from build123d import *

# Parameters (mm, degrees)
BOSS_EXTRUDE1_DEPTH     = 70
CUT_EXTRUDE2_DEPTH      = 83.5
CUT_EXTRUDE2_DEPTH_BACK = 83.5


with BuildPart() as part:
    # Sketch1 → Boss-Extrude1 (new body)
    with BuildSketch(Plane(origin=(0, 0, 0), x_dir=(1, 0, 0), z_dir=(0, 1, 0))):
        Polygon((-42.5, 0), (42.5, 0), (42.5, 10), (41.5, 10), (41.5, 1), (-41.5, 1), (-41.5, 10), (-42.5, 10), align=None)
    extrude(amount=BOSS_EXTRUDE1_DEPTH)

    # Sketch2 → Cut-Extrude2 (cut, two sides: drawn at the far end of the back side and taken through both)
    with BuildSketch(Plane(origin=(0, 0, 0), x_dir=(0, 0, -1), z_dir=(1, 0, 0)).offset(-CUT_EXTRUDE2_DEPTH_BACK)):
        Polygon((1, 70), (10, 55), (10, 70), align=None)
    extrude(amount=CUT_EXTRUDE2_DEPTH + CUT_EXTRUDE2_DEPTH_BACK, mode=Mode.SUBTRACT)


solid = part.part
Geometry check sheet. Reference: the model listing, model coordinates, mm. A direction names the side the tool comes from. Round coordinates to 2 decimals unless told otherwise and drop trailing zeros. Write each loop counter-clockwise with the first axis right and the second up, starting at its lowest first coordinate (ties: lowest second). Pieces come first, ordered by that corner, then holes. Notation, with made-up numbers: (46, -9) -> (67, -9) arc R13 ccw to (67, 4) -> close; hole circle Ø3 at (88, 59.5). An arc over 180 degrees is marked (long way). One line per item, written item: value. Start each with the question number.
(1) Draft check along X on faces 1 (the flat face through (-42.5, 35, -5)), 2 (the flat face through (1, 35, -1)), 3 (the flat face through (41.99, 62.6, -5.44)). Enter one of: +X half, -X half, draft (parallel to the pull), parting line (faces both ways), or undercut.
(2) Access from +Z, -Z, +X, -X, +Y, -Y to the whole of each face (thin tool, end or side, straight path). Record for faces 4 (the flat face through (-1, 35, 0)), 5 (the flat face through (-41.5, 35, -5)).
(3) Cross-section at D-D, the plane z = -8.25. Record the cut outline in (x, y), and give its area (3 significant figures).
(4) Cross-section at B-B, the plane y = 51. Record the cut outline in (x, z).
(5) Scan lines: line 1 (X direction, y = 48.5, z = -7); line 2 (Z direction, x = -9.5, y = 33.5). Record each from-to range of solid material in increasing order. Write a range as [from, to].
(6) Go/stop test with a flat-tipped pin: pin 1 Ø6 at (x, y) = (12.5, 53.5) entering from -Z. Record where the tip stops, or that it passes through.
(7) Cross-section at A-A, the plane z = -2.5. Record the cut outline in (x, y), and give its area (3 significant figures).
(8) Cross-section at C-C, the plane y = 60.5. Record the cut outline in (x, z).
Answer:
1. face 1: -X half
1. face 2: undercut
1. face 3: draft
2. face 4: +Z, +X, -X, +Y, -Y
2. face 5: -Z, +Y, -Y
3. outline: (-42.5, 0) -> (-41.5, 0) -> (-41.5, 57.92) -> (-42.5, 57.92) -> close; (41.5, 0) -> (42.5, 0) -> (42.5, 57.92) -> (41.5, 57.92) -> close
3. area: 116 mm²
4. outline: (-42.5, -10) -> (-41.5, -10) -> (-41.5, -1) -> (41.5, -1) -> (41.5, -10) -> (42.5, -10) -> (42.5, 0) -> (-42.5, 0) -> close
5. line 1: [-42.5, -41.5], [41.5, 42.5]
5. line 2: [-1, 0]
6. pin 1: z = -1
7. outline: (-42.5, 0) -> (-41.5, 0) -> (-41.5, 67.5) -> (-42.5, 67.5) -> close; (41.5, 0) -> (42.5, 0) -> (42.5, 67.5) -> (41.5, 67.5) -> close
7. area: 135 mm²
8. outline: (-42.5, -6.7) -> (-41.5, -6.7) -> (-41.5, -1) -> (41.5, -1) -> (41.5, -6.7) -> (42.5, -6.7) -> (42.5, 0) -> (-42.5, 0) -> close
